Could you check a few things on this model? Use its own coordinates, in mm. Face numbers are marked on the shaded views. Round coordinates to 2 decimals unless told otherwise and drop trailing zeros. Write each loop counter-clockwise with the first axis right and the second up, starting at its lowest first coordinate (ties: lowest second). Pieces come first, ordered by that corner, then holes. Notation, with made-up numbers: (17.5, 18) - (74.5, 18) arc R21 ccw to (74.5, 37) - close; hole circle Ø4 at (53.5, 67.25). An arc over 180 degrees is marked (long way). Write each question's results on one line, items separated by ' | '. Start each with the question number.
(1) For P1, Ø1.5, axis at x = -25.5, z = -1.5, coming from the +Y side, with a flat end and sliding along its axis, tell me the tip position at first contact or that it passes through.
(2) Thinking about a two-plate mould opening in Z: for the marked faces 1, 2 and 3, which applies, +Z half, -Z half, draft (parallel to the pull), parting line (faces both ways), or undercut?
(3) Imagine slicing it at A-A on x = 0. Write out the boundary of the cut face in (y, z), then the cut area to 3 significant figures.
(4) Please list where these lines run through material, in increasing order: line 1 (Y direction, x = 0, z = -6.25); line 2 (Y direction, x = 0, z = -0.95); line 3 (Z direction, x = 39.5, y = 8.5). Write a range as [from, to].
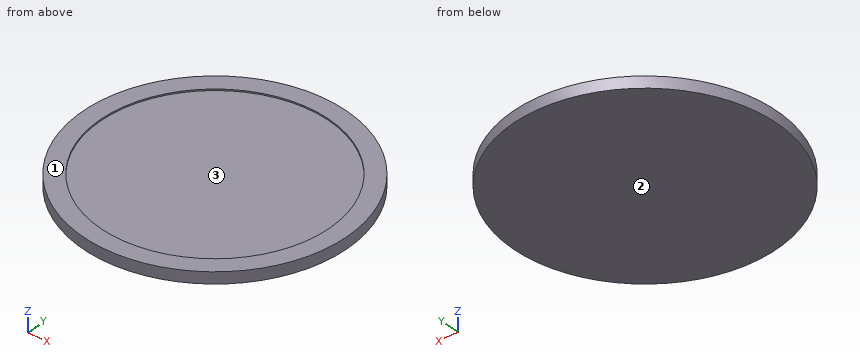
```python
from build123d import *

# Parameters (mm, degrees)
SKETCH040_R   = 92.3
SKETCH040_R_2 = 80
PAD025_DEPTH  = 1
SKETCH041_R   = 92.3
SKETCH041_R_2 = 90
PAD026_DEPTH  = 5
FILLET_R      = 4
SKETCH042_R   = 92.3
PAD027_DEPTH  = 2


with BuildPart() as part:
    # Sketch040 → Pad025 (new body)
    with BuildSketch(Plane.XY):
        Circle(SKETCH040_R)
        Circle(SKETCH040_R_2, mode=Mode.SUBTRACT)
    extrude(amount=PAD025_DEPTH)

    # Sketch041 (on Face3 of Pad025) → Pad026 (join)
    with BuildSketch(Plane(origin=(0, 0, 0), x_dir=(1, 0, 0), z_dir=(0, 0, -1))):
        Circle(SKETCH041_R)
        Circle(SKETCH041_R_2, mode=Mode.SUBTRACT)
    extrude(amount=PAD026_DEPTH)

    # Fillet
    fillet_edges = [part.edges().sort_by_distance(p)[0] for p in [
        (-90, 0, 0),
    ]]
    fillet(fillet_edges, radius=FILLET_R)

    # Sketch042 (on Face3 of Fillet) → Pad027 (join)
    with BuildSketch(Plane(origin=(0, 0, -5), x_dir=(1, 0, 0), z_dir=(0, 0, -1))):
        Circle(SKETCH042_R)
    extrude(amount=PAD027_DEPTH)


with BuildPart() as part_1:
    # Body025 placement: moved
    add(part.part.moved(Location((0, 0, -1.6))))


solid = part_1.part
```
Response:
1) P1: y = 88.92
2) face 1: +Z half | face 2: -Z half | face 3: undercut
3) outline: (-92.3, -8.6) - (92.3, -8.6) - (92.3, -0.6) - (80, -0.6) - (80, -1.6) - (86, -1.6) arc R4 cw to (90, -5.6) - (90, -6.6) - (-90, -6.6) - (-90, -5.6) arc R4 cw to (-86, -1.6) - (-80, -1.6) - (-80, -0.6) - (-92.3, -0.6) - close | area: 424 mm²
4) line 1: [-92.3, -90], [90, 92.3] | line 2: [-92.3, -80], [80, 92.3] | line 3: [-8.6, -6.6]
